```python
from build123d import *

# Parameters (mm, degrees)
SKETCH1_W                                      = 44.45
SKETCH1_H                                      = 38.1
BOSS_EXTRUDE1_DEPTH                            = 6.35
CSK_FOR_4_FLAT_HEAD_MACHINE_SCREW1_D           = 3.2639
CSK_FOR_4_FLAT_HEAD_MACHINE_SCREW1_CSINK_D     = 5.715
CSK_FOR_4_FLAT_HEAD_MACHINE_SCREW1_CSINK_ANGLE = 82
SKETCH4_R                                      = 4.7625
BOSS_EXTRUDE2_DEPTH                            = 3.175
FILLET2_R                                      = 6.858
FILLET3_R                                      = 6.35


with BuildPart() as part:
    # Sketch1 → Boss-Extrude1 (new body)
    with BuildSketch(Plane.XY):
        Rectangle(SKETCH1_W, SKETCH1_H)
    extrude(amount=BOSS_EXTRUDE1_DEPTH)

    # CSK for #4 Flat Head Machine Screw1 (through all)
    with Locations(Plane.XY.offset(6.35)):
        with Locations((-19.05, 12.7), (19.05, -12.7), (-19.05, -12.7), (19.05, 12.7)):
            CounterSinkHole(CSK_FOR_4_FLAT_HEAD_MACHINE_SCREW1_D / 2, CSK_FOR_4_FLAT_HEAD_MACHINE_SCREW1_CSINK_D / 2, counter_sink_angle=CSK_FOR_4_FLAT_HEAD_MACHINE_SCREW1_CSINK_ANGLE)

    # Sketch4 → Boss-Extrude2 (add, symmetric)
    with BuildSketch(Plane(origin=(0, 0, 0), x_dir=(1, 0, 0), z_dir=(0, 1, 0))):
        with BuildLine():
            Line((-12.341914895, -56.026561414), (-22.225, -6.35))
            Line((-22.225, -6.35), (22.225, -6.35))
            Line((22.225, -6.35), (6.07586016, -57.058395803))
            ThreePointArc((6.07586016, -57.058395803), (-3.532791524, -63.678087179), (-12.341914895, -56.026561414))
        make_face()
        with Locations(Location((-2.99999997, -54.168, 0), (0, 0, 270))):
            Circle(SKETCH4_R, mode=Mode.SUBTRACT)
    extrude(amount=BOSS_EXTRUDE2_DEPTH, both=True)

    # Fillet2
    fillet2_edges = [part.edges().sort_by_distance(p)[0] for p in [
        (22.225, -19.05, 3.175),
        (-22.225, -19.05, 3.175),
        (-22.225, 19.05, 3.175),
        (22.225, 19.05, 3.175),
    ]]
    fillet(fillet2_edges, radius=FILLET2_R)

    # Fillet3
    # the kernel refuses this fillet: 6.35 mm, written as the material it adds along each edge
    with BuildSketch(Plane(origin=(-22.225, 3.175, 6.35), x_dir=(0, 1, 0), z_dir=(1, 0, 0))) as fillet3_piece_1_section:
        with BuildLine():
            CenterArc((FILLET3_R, FILLET3_R), FILLET3_R, 180, 90)
            Line((0, FILLET3_R), (0, 0))
            Line((0, 0), (FILLET3_R, 0))
        make_face()
    fillet3_piece_1 = extrude(amount=44.45, mode=Mode.PRIVATE)
    fillet3_piece_1 = split(fillet3_piece_1, bisect_by=Plane(origin=(-21.111154549, 4.625615872, 11.948657846), z_dir=(0.980778469831864, 0, -0.19512455794765435)), keep=Keep.TOP, mode=Mode.PRIVATE)
    fillet3_piece_1 = split(fillet3_piece_1, bisect_by=Plane(origin=(19.761324723, 4.625615872, 14.085955123), z_dir=(-0.9528462078877957, 0, -0.30345362761688605)), keep=Keep.TOP, mode=Mode.PRIVATE)
    add(fillet3_piece_1)
    with BuildSketch(Plane(origin=(-22.225, -3.175, 6.35), x_dir=(0, -1, 0), z_dir=(1, 0, 0))) as fillet3_piece_2_section:
        with BuildLine():
            CenterArc((FILLET3_R, -FILLET3_R), FILLET3_R, 90, 90)
            Line((0, -FILLET3_R), (0, 0))
            Line((0, 0), (FILLET3_R, 0))
        make_face()
    fillet3_piece_2 = extrude(amount=44.45, mode=Mode.PRIVATE)
    fillet3_piece_2 = split(fillet3_piece_2, bisect_by=Plane(origin=(-21.111154549, -4.625615872, 11.948657846), z_dir=(0.980778469831864, 0, -0.19512455794765435)), keep=Keep.TOP, mode=Mode.PRIVATE)
    fillet3_piece_2 = split(fillet3_piece_2, bisect_by=Plane(origin=(19.761324723, -4.625615872, 14.085955123), z_dir=(-0.9528462078877957, 0, -0.30345362761688605)), keep=Keep.TOP, mode=Mode.PRIVATE)
    add(fillet3_piece_2)


solid = part.part
```
Could you check a few things on this model? Use its own coordinates, in mm. A direction names the side the tool comes from. Give positions to 0.01 mm unless a question says otherwise; leave off trailing zeros. Loops run counter-clockwise (first coordinate to the right, second up) from the corner with the lowest first, then second, coordinate; pieces in that order, holes last. Notation, with made-up numbers: (36.25, -38) - (54.25, -38) arc R24 ccw to (54.25, -21) - close; hole circle Ø8 at (28, -20). An arc over 180 degrees is marked (long way). Answer in a Markdown table with one row per item. Add a question column.
Q1. Which directions (+Z, -Z, +X, -X, +Y, -Y) give clear straight access to the entire face, cutting with the end or side of a thin tool? Please do faces 5 (the face through (0, 3.175, 32)), 6 (the face through (-20.269, -16.988, 3.219)).
Q2. For pin 1 (1 mm diameter, centred on x = 16.5, z = 32, fed in from -Y); pin 2 (20.5 mm diameter, centred on x = -5.5, z = 37, fed in from -Y) (3 decimals); pin 3 (5 mm diameter, centred on x = -2, y = 13, fed in from +Z); pin 4 (20.5 mm diameter, centred on x = 4.5, z = 28, fed in from +Y) (3 decimals), each with a flat end and sliding along its axis, tell me the tip position at first contact or that it passes through.
Q3. Please list where these lines run through material, in increasing order: L1, parallel to Y at x = -19, z = 1; L2, parallel to X at y = -12.7, z = 2.75; L3, parallel to Z at x = 15.5, y = 14. Write a range as from..to.
Q4. If we section it at D-D (x = -19.05): State how many separate pieces and enclosed holes the cut face has, plus the area to 3 significant figures.
Q5. If we section it at C-C (z = 51): List the corners of the cut face in (x, y) for me (3 decimals), plus the area to 3 significant figures.
Q6. We'd pull the mould along Z, two halves only. Please class faces 1 (the face through (0, 19.05, 3)), 2 (the face through (0, 0, 0)), 3 (the face through (-2.79, -0.04, 49.41)), 4 (the face through (0, 14, 6.35)): +Z half, -Z half, draft (parallel to the pull), parting line (faces both ways), or undercut.
The answers:
| question | item | result |
|---|---|---|
| 1 | face 5 | +Z, +X, -X, +Y |
| 1 | face 6 | +Z, -Z, -X, -Y |
| 2 | pin 1 | passes through |
| 2 | pin 2 | stops at y = -3.175 |
| 2 | pin 3 | stops at z = 6.35 |
| 2 | pin 4 | stops at y = 3.175 |
| 3 | L1 | y = -18.01..-14.33, -11.07..11.07, 14.33..18.01 |
| 3 | L2 | x = -22.21..-20.68, -17.42..17.42, 20.68..22.21 |
| 3 | L3 | z = 0..6.35 |
| 4 | separate pieces | 3 |
| 4 | enclosed holes | 0 |
| 4 | area | 302 mm^2 |
| 5 | outline | (-13.342, -3.175) - (-6.556, -3.175) - (-6.556, 3.175) - (-13.342, 3.175) - close; (0.556, -3.175) - (8.005, -3.175) - (8.005, 3.175) - (0.556, 3.175) - close |
| 5 | area | 90.4 mm^2 |
| 6 | face 1 | draft |
| 6 | face 2 | -Z half |
| 6 | face 3 | undercut |
| 6 | face 4 | +Z half |
